Build history of the part. All positions in model axes, mm. Round coordinates to 2 decimals unless told otherwise and drop trailing zeros. Write each loop counter-clockwise with the first axis right and the second up, starting at its lowest first coordinate (ties: lowest second). Pieces come first, ordered by that corner, then holes. Notation, with made-up numbers: (59, 61.5) - (104, 61.5) arc R23 ccw to (104, 88.5) - close; hole circle Ø5 at (-25, 17). An arc over 180 degrees is marked (long way). Answer as a JSON object with one key per item and string values. Group by question number.
Item 1: Slice it at D-D, the plane x = -51. List the corners of the cut face in (y, z) (3 decimals).
Item 2: Slice it at C-C, the plane x = -120.65. List the corners of the cut face in (y, z) (3 decimals).
Item 3: Probe line 1 (Y direction, x = -120.65, z = 0.7) (3 decimals); line 2 (X direction, y = 68.5, z = 2.75); line 3 (X direction, y = -61, z = 2.5). List the from-to ranges inside material, lowest first. Write a range as from..to.
Item 4: Slice it at A-A, the plane y = 0. List the corners of the cut face in (x, z) (3 decimals).
Item 5: Slice it at B-B, the plane z = 0.85. List the corners of the cut face in (x, y) (3 decimals).
Item 6: Flat gauge pins, fed straight in: pin 1 (1 mm diameter, centred on x = -60, z = 1.5, fed in from +Y); pin 2 (1 mm diameter, centred on x = -135.5, z = 2, fed in from -Y). Where does each tip first touch, or does it go through?
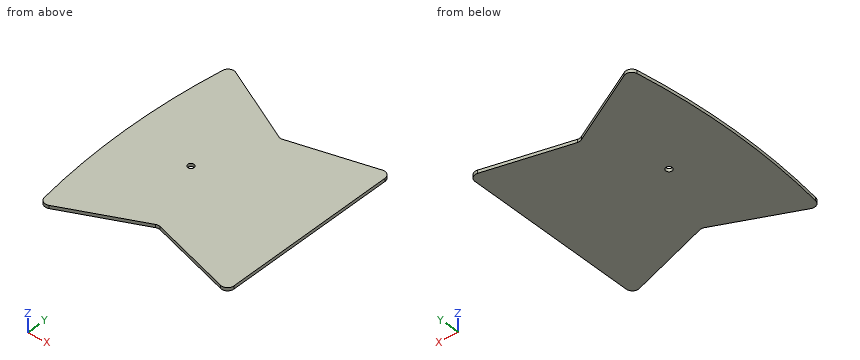
from build123d import *

# Parameters (mm, degrees)
SKETCH1_R           = 3.175
BOSS_EXTRUDE1_DEPTH = 3.175
FILLET1_R           = 6.35


with BuildPart() as part:
    # Sketch1 → Boss-Extrude1 (new body)
    with BuildSketch(Plane.XY):
        with BuildLine():
            Line((-177.8, 111.125), (-91.8765625, 69.85))
            Line((-91.8765625, 69.85), (0, 95.25))
            Line((0, 95.25), (0, -95.25))
            Line((0, -95.25), (-91.8765625, -69.85))
            Line((-91.8765625, -69.85), (-177.8, -111.125))
            ThreePointArc((-177.8, -111.125), (-186.948920727, 0), (-177.8, 111.125))
        make_face()
        with Locations((-120.65, 0)):
            Circle(SKETCH1_R, mode=Mode.SUBTRACT)
    extrude(amount=BOSS_EXTRUDE1_DEPTH)

    # Fillet1
    fillet1_edges = [part.edges().sort_by_distance(p)[0] for p in [
        (-177.8, 111.125, 1.5875),
        (-91.8765625, 69.85, 1.5875),
        (0, 95.25, 1.5875),
        (0, -95.25, 1.5875),
        (-91.8765625, -69.85, 1.5875),
        (-177.8, -111.125, 1.5875),
    ]]
    fillet(fillet1_edges, radius=FILLET1_R)


solid = part.part
Geometry says:
{
 "1": {"outline": "(-81.151, 0) - (81.151, 0) - (81.151, 3.175) - (-81.151, 3.175) - close"},
 "2": {"outline": "(-83.672, 0) - (-3.175, 0) - (-3.175, 3.175) - (-83.672, 3.175) - close; (3.175, 0) - (83.672, 0) - (83.672, 3.175) - (3.175, 3.175) - close"},
 "3": {"line 1": "y = -83.672..-3.175, 3.175..83.672", "line 2": "x = -183.49..0", "line 3": "x = -184.21..0"},
 "4": {"outline": "(-186.949, 0) - (-123.825, 0) - (-123.825, 3.175) - (-186.949, 3.175) - close; (-117.475, 0) - (0, 0) - (0, 3.175) - (-117.475, 3.175) - close"},
 "5": {"outline": "(-179.147, -102.672) arc R6.35 ccw to (-170.12, -107.436) - (-94.023, -70.881) arc R6.35 cw to (-89.581, -70.485) - (-8.042, -93.027) arc R6.35 ccw to (0, -86.906) - (0, 86.906) arc R6.35 ccw to (-8.042, 93.027) - (-89.581, 70.485) arc R6.35 cw to (-94.023, 70.881) - (-170.12, 107.436) arc R6.35 ccw to (-179.147, 102.672) arc R679.45 ccw to start; hole circle Ø6.35 at (-120.65, 0)"},
 "6": {"pin 1": "stops at y = 78.8", "pin 2": "stops at y = -91.05"}
}
